```python
from build123d import *

# Parameters (mm, degrees)
F0_W     = 30
F0_H     = 19
F1_DEPTH = 4
F2_R     = 2.25
F3_DEPTH = 25
F4_W     = 10
F4_H     = 11
F5_DEPTH = 11.9
F6_R     = 3.3
F7_DEPTH = 25
F8_R     = 1


with BuildPart() as f1:
    # F0 (on Front) → F1 (new body)
    with BuildSketch(Plane.XZ):
        with Locations((15, 9.5)):
            Rectangle(F0_W, F0_H)
    extrude(amount=F1_DEPTH)

    # F2 (on face) → F3 (cut)
    with BuildSketch(Plane.XZ.offset(4)):
        with Locations((25, 9.5)):
            Circle(F2_R)
        with Locations((5, 9.5)):
            Circle(F2_R)
    extrude(amount=-F3_DEPTH, mode=Mode.SUBTRACT)

    # F4 (on face) → F5 (join)
    with BuildSketch(Plane.XZ.offset(4)):
        with Locations((15, 8.5)):
            Rectangle(F4_W, F4_H)
    extrude(amount=F5_DEPTH)

    # F6 (on face) → F7 (cut)
    with BuildSketch(Plane.XY.offset(14)):
        with Locations((15, -10)):
            Circle(F6_R)
    extrude(amount=-F7_DEPTH, mode=Mode.SUBTRACT)

    # F8
    f8_edges = [f1.edges().sort_by_distance(p)[0] for p in [
        (0, -2, 19),
        (30, -2, 19),
        (30, -2, 0),
        (0, -2, 0),
    ]]
    fillet(f8_edges, radius=F8_R)


solid = f1.part
```
Check sheet for the modelled part. Datum: model origin and axes. Units: mm. A direction names the side the tool comes from. Round coordinates to 2 decimals unless told otherwise and drop trailing zeros. Loops run counter-clockwise (first coordinate to the right, second up) from the corner with the lowest first, then second, coordinate; pieces in that order, holes last. Notation, with made-up numbers: (40, 12.5) -> (69, 12.5) arc R28 ccw to (69, 44.5) -> close; hole circle Ø5 at (-37.5, 29.5). An arc over 180 degrees is marked (long way). Write item = value, one per line. Start each with the question number.
1) Sectioned sample at B-B, the plane y = -2.25. Record the cut outline in (x, z).
2) Sectioned sample at D-D, the plane z = 6.75. Record the cut outline in (x, y), plus the area to 3 significant figures.
3) Sectioned sample at A-A, the plane z = 9.5. Record the cut outline in (x, y).
4) Sectioned sample at C-C, the plane x = 5. Record the cut outline in (y, z).
5) Thickness scan on probe 1 along Z at (x, y) = (25, -2.5); probe 2 along Y at (x, z) = (15, 7.75); probe 3 along X at (y, z) = (-3.5, 9.25). Record the ranges inside material, lowest first.
6) Gauge pin test, flat ends, axial feed: pin 1 Ø5 at (x, y) = (17, -11.5) entering from -Z; pin 2 Ø3.5 at (y, z) = (-13, 10.5) entering from +X; pin 3 Ø3 at (y, z) = (-7, 4) entering from -X; pin 4 Ø2.5 at (x, z) = (25, 9.5) entering from +Y. Record the tip position at first contact, or that the pin passes through.
7) Set-up check for faces 5 (the flat face through (13, -7, 14)), 6 (the flat face through (20, -10, 8)), 7 (the flat face through (30, -2, 9)), 8 (the flat face through (13, -7, 3)), 9 (the flat face through (10, -10, 8)): record each of +Z, -Z, +X, -X, +Y, -Y from which the full face is reachable in a straight line by a thin tool's end or side.
8) Release check for a two-part mould opening along Z. For faces 1 (the cylindrical face through (27.146, -2.028, 10.176)), 2 (the cylindrical face through (0.285, -2.028, 0.301)), 3 (the cylindrical face through (6.21, -2.028, 11.397)), 4 (the cylindrical face through (29.699, -2.028, 18.715)) record: released by +Z, released by -Z, zero draft, split by the parting line, or undercut.
Results are:
q1.outline = (0, 1) arc R1 ccw to (1, 0) -> (29, 0) arc R1 ccw to (30, 1) -> (30, 18) arc R1 ccw to (29, 19) -> (1, 19) arc R1 ccw to (0, 18) -> close; hole circle Ø4.5 at (5, 9.5); hole circle Ø4.5 at (25, 9.5)
q2.outline = (0, -4) -> (10, -4) -> (10, -15.9) -> (20, -15.9) -> (20, -4) -> (30, -4) -> (30, 0) -> (0, 0) -> close; hole circle Ø6.6 at (15, -10)
q2.area = 205 mm^2
q3.outline = (0, -4) -> (2.75, -4) -> (2.75, 0) -> (0, 0) -> close; (7.25, -4) -> (10, -4) -> (10, -15.9) -> (20, -15.9) -> (20, -4) -> (22.75, -4) -> (22.75, 0) -> (7.25, 0) -> close; (27.25, -4) -> (30, -4) -> (30, 0) -> (27.25, 0) -> close; hole circle Ø6.6 at (15, -10)
q4.outline = (-4, 0) -> (0, 0) -> (0, 7.25) -> (-4, 7.25) -> close; (-4, 11.75) -> (0, 11.75) -> (0, 19) -> (-4, 19) -> close
q5.probe_1 = 0 to 7.25, 11.75 to 19
q5.probe_2 = -15.9 to -13.3, -6.7 to 0
q5.probe_3 = 0 to 2.76, 7.24 to 22.76, 27.24 to 30
q6.pin_1 = 3
q6.pin_2 = 20
q6.pin_3 = 10
q6.pin_4 = through
q7.face_5 = +Z, +X, -X, -Y
q7.face_6 = +Z, -Z, +X, -Y
q7.face_7 = +Z, -Z, +X, +Y, -Y
q7.face_8 = -Z, +X, -X, -Y
q7.face_9 = +Z, -Z, -X, -Y
q8.face_1 = undercut
q8.face_2 = released by -Z
q8.face_3 = undercut
q8.face_4 = released by +Z
